The model under review builds one solid part; all positions refer to its coordinate system, in mm. Round coordinates to 2 decimals unless told otherwise and drop trailing zeros. Write each loop counter-clockwise with the first axis right and the second up, starting at its lowest first coordinate (ties: lowest second). Pieces come first, ordered by that corner, then holes. Notation, with made-up numbers: (-33, 72) - (-7, 72) arc R30 ccw to (-7, 107) - close; hole circle Ø1 at (-8.75, 54.25). An arc over 180 degrees is marked (long way). Write each question's results on one line, items separated by ' | '.
```python
from build123d import *

# Parameters (mm, degrees)
SKETCH1_R               = 7.94
SKETCH1_R_2             = 6.44
BOSS_EXTRUDE1_DEPTH     = 70.91
CHAMFER1_SIZE           = 0.25
SKETCH2_R               = 1.55
CUT_EXTRUDE1_DEPTH      = 5.405594573
CUT_EXTRUDE1_DEPTH_BACK = 17.105594573


with BuildPart() as part:
    # Sketch1 → Boss-Extrude1 (new body)
    with BuildSketch(Plane(origin=(0, 0, 0), x_dir=(1, 0, 0), z_dir=(0, 1, 0))):
        Circle(SKETCH1_R)
        Circle(SKETCH1_R_2, mode=Mode.SUBTRACT)
    extrude(amount=BOSS_EXTRUDE1_DEPTH)

    # Chamfer1
    chamfer1_edges = [part.edges().sort_by_distance(p)[0] for p in [
        (-7.94, 0, 0),
        (-7.94, 70.91, 0),
    ]]
    chamfer(chamfer1_edges, length=CHAMFER1_SIZE)

    # Sketch2 → Cut-Extrude1 (cut, two sides)
    with BuildSketch(Plane(origin=(-2.093493753, 0, 5.462580334), x_dir=(0.933774416, 0, 0.35786218), z_dir=(-0.35786218, 0, 0.933774416))) as cut_extrude1_sk:
        with Locations((0, 63.41)):
            Circle(SKETCH2_R)
        with Locations((0, 7.5)):
            Circle(SKETCH2_R)
    extrude(amount=CUT_EXTRUDE1_DEPTH, mode=Mode.SUBTRACT)
    extrude(cut_extrude1_sk.sketch, amount=-CUT_EXTRUDE1_DEPTH_BACK, mode=Mode.SUBTRACT)


solid = part.part
```
Q1. We need section B-B (z = 0). State the section outline as (x, y) points, plus the area to 3 significant figures.
Evaluation:
outline: (-7.94, 0.25) - (-7.69, 0) - (-6.44, 0) - (-6.44, 70.91) - (-7.69, 70.91) - (-7.94, 70.66) - close; (6.44, 0) - (7.69, 0) - (7.94, 0.25) - (7.94, 70.66) - (7.69, 70.91) - (6.44, 70.91) - close | area: 213 mm^2
Q2. The part is to be moulded in two halves that separate along Y. For faces 1 (the cylindrical face through (1.386, 62.467, -7.054)), 2 (the flat face through (-5, 70.91, 5)), 3 (the flat face through (-5, 0, 5)), say which applies: released by +Y, released by -Y, zero draft, split by the parting line, or undercut.
Evaluation:
face 1: undercut | face 2: released by +Y | face 3: released by -Y
Q3. We need section D-D (x = -2.75). State how many separate pieces and enclosed holes the cut face has, plus the area to 3 significant figures.
Evaluation:
separate pieces: 4 | enclosed holes: 0 | area: 220 mm^2
Q4. For probe 1 along X at (y, z) = (23.5, 0); probe 2 along X at (y, z) = (25.5, -4), list the stretches that pass through material, from the lowest coordinate up.
Evaluation:
probe 1: x = -7.94 to -6.44, 6.44 to 7.94 | probe 2: x = -6.86 to -5.05, 5.05 to 6.86
Q5. Insertion check: P1, Ø8, axis at x = -4.5, y = 40, coming from the -Z side; P2, Ø1, axis at y = 21.5, z = -4.5, coming from the -X side; P3, Ø4, axis at x = 5, y = 16.5, coming from the -Z side. Each pin has a flat end and moves straight along its axis. Give the tip position at first contact, or say it passes through.
Evaluation:
P1: stops at z = -7.92 | P2: stops at x = -6.86 | P3: stops at z = -7.35
Q6. We need section C-C (y = 33). State the section outline as (x, z) points, plus the area to 3 significant figures.
Evaluation:
outline: circle Ø15.88 at (0, 0); hole circle Ø12.88 at (0, 0) | area: 67.8 mm^2
Q7. We need section A-A (x = 0). State the section outline as (y, z) points.
Evaluation:
outline: (0, -7.69) - (0.25, -7.94) - (70.66, -7.94) - (70.91, -7.69) - (70.91, -6.44) - (0, -6.44) - close; (0, 6.44) - (70.91, 6.44) - (70.91, 7.69) - (70.66, 7.94) - (0.25, 7.94) - (0, 7.69) - close
